The listing builds one solid part. Answer for the finished solid, in the listing's coordinates (mm). A direction names the side the tool comes from. Round coordinates to 2 decimals unless told otherwise and drop trailing zeros. Write each loop counter-clockwise with the first axis right and the second up, starting at its lowest first coordinate (ties: lowest second). Pieces come first, ordered by that corner, then holes.
from build123d import *

# Parameters (mm, degrees)
SKICA2_W                 = 50
SKICA2_H                 = 50
P_IDAT_VYSUNUT_M1_DEPTH  = 25
SKICA3_W                 = 20.588514008
SKICA3_H                 = 12.517673613
ODEBRAT_VYSUNUT_M1_DEPTH = 39
SKICA4_W                 = 14.884932554
SKICA4_H                 = 9.667623342
ODEBRAT_VYSUNUT_M2_DEPTH = 39
SKICA5_W                 = 16.426867347
SKICA5_H                 = 18.535662784
ODEBRAT_VYSUNUT_M3_DEPTH = 39


with BuildPart() as part:
    # Skica2 → Přidat vysunutím1 (new body, symmetric)
    with BuildSketch(Plane.XY):
        with Locations((25, 25)):
            Rectangle(SKICA2_W, SKICA2_H)
    extrude(amount=P_IDAT_VYSUNUT_M1_DEPTH, both=True)

    # Skica3 → Odebrat vysunutím1 (cut)
    with BuildSketch(Plane(origin=(0, 50, 0), x_dir=(1, 0, 0), z_dir=(0, 1, 0))):
        with Locations((29.470091853, -18.741163194)):
            Rectangle(SKICA3_W, SKICA3_H)
    extrude(amount=-ODEBRAT_VYSUNUT_M1_DEPTH, mode=Mode.SUBTRACT)

    # Skica4 → Odebrat vysunutím2 (cut)
    with BuildSketch(Plane(origin=(50, 0, 0), x_dir=(0, 0, -1), z_dir=(1, 0, 0))):
        with Locations((0.371136043, 4.833811671)):
            Rectangle(SKICA4_W, SKICA4_H)
    extrude(amount=-ODEBRAT_VYSUNUT_M2_DEPTH, mode=Mode.SUBTRACT)

    # Skica5 → Odebrat vysunutím3 (cut)
    with BuildSketch(Plane.ZY):
        with Locations((-16.786566327, 34.267831392)):
            Rectangle(SKICA5_W, SKICA5_H)
    extrude(amount=-ODEBRAT_VYSUNUT_M3_DEPTH, mode=Mode.SUBTRACT)


solid = part.part
1. Section D-D on x = 26 is taken. Determine the outline of the cut face in (y, z), plus the area to 3 significant figures.
Geometry says:
outline: (0, -25) - (25, -25) - (25, -8.57) - (43.54, -8.57) - (43.54, -25) - (50, -25) - (50, 12.48) - (11, 12.48) - (11, 25) - (0, 25) - (0, 7.07) - (9.67, 7.07) - (9.67, -7.81) - (0, -7.81) - close
area: 1,560 mm2
2. A tool of negligible diameter and unlimited length cuts with its end or side. For faces 1 (the face through (30, 20, -25)), 2 (the face through (31, 9.668, 0)), 3 (the face through (19, 25, -17)), 4 (the face through (29, 11, 19)), from which of +Z, -Z, +X, -X, +Y, -Y can it reach the whole face along a straight path? Write none if from no direction.
Geometry says:
face 1: -Z, +X, -X, +Y, -Y
face 2: +X, -Y
face 3: -Z, -X
face 4: +Z, +Y
3. Straight lines are drawn through the part: line 1 along X through (y, z) = (41, 14.5); line 2 along Z through (x, y) = (22.5, 3.5); line 3 along Y through (x, z) = (9.5, -21). For each, find the intervals that lie inside material, in ascending order.
Geometry says:
line 1: x = 0 to 19.18, 39.76 to 50
line 2: z = -25 to -7.81, 7.07 to 25
line 3: y = 0 to 25, 43.54 to 50
4. Section A-A on y = 26 is taken. Determine the outline of the cut face in (x, z), plus the area to 3 significant figures.
Geometry says:
outline: (0, -8.57) - (39, -8.57) - (39, -25) - (50, -25) - (50, 25) - (39.76, 25) - (39.76, 12.48) - (19.18, 12.48) - (19.18, 25) - (0, 25) - close
area: 1,600 mm2
5. Section C-C on z = 22 is taken. Determine the outline of the cut face in (x, y).
Geometry says:
outline: (0, 0) - (50, 0) - (50, 50) - (39.76, 50) - (39.76, 11) - (19.18, 11) - (19.18, 50) - (0, 50) - close
6. Given pin 1 (5 mm diameter, centred on x = 8.5, y = 28.5, fed in from -Z); pin 2 (10 mm diameter, centred on x = 28, z = 21, fed in from +Y); pin 3 (5 mm diameter, centred on y = 6, z = 2.5, fed in from +X), each flat-ended and moving along its own axis, determine where each tip first touches the part or whether it passes through.
Geometry says:
pin 1: stops at z = -8.57
pin 2: stops at y = 11
pin 3: stops at x = 11
7. For a pull along Z with two mould halves and no side action, classify faces 5 (the face through (29, 31, 12.482)), 6 (the face through (25, 0, 11)), 7 (the face through (11, 5, 0)) as released by +Z, released by -Z, zero draft, split by the parting line, or undercut.
Geometry says:
face 5: released by +Z
face 6: zero draft
face 7: undercut
8. Section B-B on x = 7 is taken. Determine the outline of the cut face in (y, z).
Geometry says:
outline: (0, -25) - (25, -25) - (25, -8.57) - (43.54, -8.57) - (43.54, -25) - (50, -25) - (50, 25) - (0, 25) - close
